from build123d import *

# Parameters (mm, degrees)
BASIC_BOX_OUTLINE_W                                = 108
BASIC_BOX_OUTLINE_H                                = 64
BASIC_BOX_OUTLINE_W_2                              = 98
BASIC_BOX_OUTLINE_H_2                              = 54
SIDE_WALLS_DEPTH                                   = 10
BOTTOM_START                                       = -2
BOTTOM_WALL_OUTLINE_W                              = 98
BOTTOM_WALL_OUTLINE_H                              = 54
BOTTOM_WALL_DEPTH                                  = 2
INNER_WALLS_TO_HOLD_DEVICES_W                      = 2
INNER_WALLS_TO_HOLD_DEVICES_H                      = 16
INSIDE_WALLS_DEPTH                                 = 10
SCREW_HOLES_R                                      = 5
SCREWS_DEPTH                                       = 10
ALIGNMENT_W                                        = 104
ALIGNMENT_H                                        = 60
ALIGNMENT_W_2                                      = 102
ALIGNMENT_H_2                                      = 58
ALIGNMENT_BUMP_DEPTH                               = 2
LEFT_START                                         = -5
LEFT_HOLE_DEPTH                                    = 5
RIGHT_HOLE_DEPTH                                   = 5
SKETCH6_W                                          = 23
SKETCH6_H                                          = 10
CUT_EXTRUDE2_DEPTH                                 = 10
CSK_FOR_10_FLAT_HEAD_MACHINE_SCREW_100_D           = 5.1054
CSK_FOR_10_FLAT_HEAD_MACHINE_SCREW_100_CSINK_D     = 9.779
CSK_FOR_10_FLAT_HEAD_MACHINE_SCREW_100_CSINK_ANGLE = 100
FILLET1_R                                          = 1.5
FILLET2_R                                          = 1.5
FILLET3_R                                          = 1


# Read off the part's stored shape, not the designer's step: bottom wall
with BuildPart() as part:
    # basic box outline → side walls (new body)
    with BuildSketch(Plane(origin=(0, 0, 0), x_dir=(1, 0, 0), z_dir=(0, 1, 0))):
        with Locations((0, 32)):
            Rectangle(BASIC_BOX_OUTLINE_W, BASIC_BOX_OUTLINE_H)
        with Locations((0, 32)):
            Rectangle(BASIC_BOX_OUTLINE_W_2, BASIC_BOX_OUTLINE_H_2, mode=Mode.SUBTRACT)
    extrude(amount=-SIDE_WALLS_DEPTH)

    # bottom wall outline → bottom wall (add)
    with BuildSketch(Plane(origin=(0, 0, 0), x_dir=(1, 0, 0), z_dir=(0, 1, 0)).offset(BOTTOM_START)):
        with Locations((0, 32)):
            Rectangle(BOTTOM_WALL_OUTLINE_W, BOTTOM_WALL_OUTLINE_H)
    extrude(amount=BOTTOM_WALL_DEPTH)

    # inner walls to hold devices → inside walls (add)
    with BuildSketch(Plane(origin=(0, 0, 0), x_dir=(1, 0, 0), z_dir=(0, 1, 0))):
        Polygon((-47, 59), (-49, 59), (-49, 55.5), (-33, 55.5), (-33, 58), (-24, 58), (-24, 54), (-14, 54), (-14, 55), (1, 55), (1, 59), (-1, 59), (-1, 57), (-16, 57), (-16, 56), (-22, 56), (-22, 59), (-35, 59), (-35, 57.5), (-47, 57.5), align=None)
        Polygon((27, 59), (25, 59), (25, 55), (40, 55), (40, 54), (49, 54), (49, 56), (42, 56), (42, 57), (27, 57), align=None)
        Polygon((49, 50), (40, 50), (40, 49), (25, 49), (25, 41), (16, 41), (16, 39), (27, 39), (27, 47), (42, 47), (42, 48), (49, 48), align=None)
        Polygon((-14, 50), (-24, 50), (-24, 46), (-33, 46), (-33, 48.5), (-35, 48.5), (-35, 21), (-33, 21), (-33, 44), (-22, 44), (-22, 48), (-16, 48), (-16, 47), (-1, 47), (-1, 39), (5, 39), (5, 41), (1, 41), (1, 49), (-14, 49), align=None)
        with Locations((-12, 13)):
            Rectangle(INNER_WALLS_TO_HOLD_DEVICES_W, INNER_WALLS_TO_HOLD_DEVICES_H)
    extrude(amount=-INSIDE_WALLS_DEPTH)

    # screw holes → screws (add)
    with BuildSketch(Plane(origin=(0, 0, 0), x_dir=(1, 0, 0), z_dir=(0, 1, 0))):
        with Locations(Location((-19, 39, 0), (0, 0, 270))):
            Circle(SCREW_HOLES_R)
        with Locations(Location((39, 39, 0), (0, 0, 270))):
            Circle(SCREW_HOLES_R)
    extrude(amount=-SCREWS_DEPTH)

    # alignment → alignment bump (add)
    with BuildSketch(Plane(origin=(0, -10, 0), x_dir=(-1, 0, 0), z_dir=(0, -1, 0))):
        with Locations((0, 32)):
            Rectangle(ALIGNMENT_W, ALIGNMENT_H)
        with Locations((0, 32)):
            Rectangle(ALIGNMENT_W_2, ALIGNMENT_H_2, mode=Mode.SUBTRACT)
    extrude(amount=ALIGNMENT_BUMP_DEPTH)

    # hole 1 → left hole (cut)
    with BuildSketch(Plane(origin=(54, 0, 0), x_dir=(0, 0, -1), z_dir=(1, 0, 0)).offset(LEFT_START)):
        with BuildLine():
            Line((46, -10), (46, -12))
            Line((46, -12), (58, -12))
            Line((58, -12), (58, -10))
            ThreePointArc((58, -10), (52, -4), (46, -10))
        make_face()
    extrude(amount=LEFT_HOLE_DEPTH, mode=Mode.SUBTRACT)

    # hole 2 → right hole (cut)
    with BuildSketch(Plane.ZY.offset(54)):
        with BuildLine():
            Line((-58, -10), (-58, -12))
            Line((-58, -12), (-46, -12))
            Line((-46, -12), (-46, -10))
            ThreePointArc((-46, -10), (-52, -4), (-58, -10))
        make_face()
    extrude(amount=-RIGHT_HOLE_DEPTH, mode=Mode.SUBTRACT)

    # Sketch6 → Cut-Extrude2 (cut)
    with BuildSketch(Plane.XY):
        with Locations((-32.5, -7)):
            Rectangle(SKETCH6_W, SKETCH6_H)
    extrude(amount=-CUT_EXTRUDE2_DEPTH, mode=Mode.SUBTRACT)

    # CSK for #10 Flat Head Machine Screw (100)1 (through all)
    with Locations(Plane(origin=(0, 0, 0), x_dir=(1, 0, 0), z_dir=(0, 1, 0))):
        with Locations((-19, 39), (39, 39)):
            CounterSinkHole(CSK_FOR_10_FLAT_HEAD_MACHINE_SCREW_100_D / 2, CSK_FOR_10_FLAT_HEAD_MACHINE_SCREW_100_CSINK_D / 2, counter_sink_angle=CSK_FOR_10_FLAT_HEAD_MACHINE_SCREW_100_CSINK_ANGLE)

    # Fillet1
    fillet1_edges = [part.edges().sort_by_distance(p)[0] for p in [
        (-52, -11, -2),
        (-52, -11, -62),
        (52, -11, -62),
        (52, -11, -2),
        (-51, -11, -61),
        (51, -11, -61),
        (51, -11, -3),
        (-51, -11, -3),
        (-54, -5, -64),
        (54, -5, -64),
        (54, -5, 0),
        (-54, -5, 0),
    ]]
    fillet(fillet1_edges, radius=FILLET1_R)

    # Fillet2
    fillet2_edges = [part.edges().sort_by_distance(p)[0] for p in [
        (0, 0, -64),
        (-54, 0, -32),
        (0, 0, 0),
        (54, 0, -32),
        (-53.560660172, 0, -0.439339828),
        (53.560660172, 0, -0.439339828),
        (53.560660172, 0, -63.560660172),
        (-53.560660172, 0, -63.560660172),
    ]]
    fillet(fillet2_edges, radius=FILLET2_R)

    # Fillet3
    # the kernel refuses this fillet: 1 mm, written as the material it adds along each edge
    with BuildSketch(Plane(origin=(-19, -2, -39), x_dir=(0, 0, 1), z_dir=(-1, 0, 0))) as fillet3_piece_1:
        with BuildLine():
            CenterArc((5 + FILLET3_R, -FILLET3_R), FILLET3_R, 90, 90)
            Line((5, -FILLET3_R), (5, 0))
            Line((5, 0), (5 + FILLET3_R, 0))
        make_face()
    revolve(axis=Axis((-19, -2, -39), (0, 1, 0)))
    with BuildSketch(Plane(origin=(39, -2, -39), x_dir=(0, 0, 1), z_dir=(-1, 0, 0))) as fillet3_piece_2:
        with BuildLine():
            CenterArc((5 + FILLET3_R, -FILLET3_R), FILLET3_R, 90, 90)
            Line((5, -FILLET3_R), (5, 0))
            Line((5, 0), (5 + FILLET3_R, 0))
        make_face()
    revolve(axis=Axis((39, -2, -39), (0, 1, 0)))


solid = part.part
Read the model definition and answer for the solid it produces. Units are mm, in the model's axes. A direction names the side the tool comes from. Give positions to 0.01 mm unless a question says otherwise; leave off trailing zeros. Loops run counter-clockwise (first coordinate to the right, second up) from the corner with the lowest first, then second, coordinate; pieces in that order, holes last. Notation, with made-up numbers: M 19,89 L 60,89 A20 ccw 60,98 Z; hole C 45,87 d5. An arc over 180 degrees is marked long. Write each question's results on one line, items separated by ' | '.
1. Straight lines are drawn through the part: line 1 (Z direction, x = 2, y = -6.75); line 2 (Z direction, x = 33.5, y = -7.5); line 3 (X direction, y = -3.5, z = -26). For each, find the intervals that lie inside material, in ascending order. Write a range as [from, to].
Values:
line 1: z = [-64, -59], [-41, -39], [-5, 0] | line 2: z = [-64, -59], [-57, -55], [-49, -47], [-5, 0] | line 3: x = [-54, -49], [-35, -33], [49, 54]
2. Section C-C on y = -7 is taken. State how many separate pieces and enclosed holes the cut face has, plus the area to 3 significant figures.
Values:
separate pieces: 7 | enclosed holes: 4 | area: 1,950 mm^2
3. The mould has two halves that part along Z. Classify faces 5 (the face through (-51, -11, -25)), 6 (the face through (52, -11, -59)): pulls with the +Z half, pulls with the -Z half, needs draft (parallel to the pull), parting line crosses it, or undercut.
Values:
face 5: undercut | face 6: needs draft
4. Section A-A on z = -26.5 is taken. Give the vertices of the cut face in (x, y).
Values:
outline: M -54,-10 L -52,-10 L -52,-12 L -51,-12 L -51,-10 L -49,-10 L -49,-2 L -35,-2 L -35,-10 L -33,-10 L -33,-2 L 49,-2 L 49,-10 L 51,-10 L 51,-12 L 52,-12 L 52,-10 L 54,-10 L 54,-1.5 A1.5 ccw 52.5,0 L -52.5,0 A1.5 ccw -54,-1.5 Z
5. Section B-B on x = -45.5 is taken. Give the vertices of the cut face in (y, z), plus the area to 3 significant figures.
Values:
outline: M -12,-62 L -10,-62 L -10,-64 L -1.5,-64 A1.5 ccw 0,-62.5 L 0,-1.5 A1.5 ccw -1.5,0 L -10,0 L -10,-2 L -12,-2 L -12,-3 L -10,-3 L -10,-5 L -2,-5 L -2,-55.5 L -10,-55.5 L -10,-57.5 L -2,-57.5 L -2,-59 L -10,-59 L -10,-61 L -12,-61 Z | area: 227 mm^2
6. Given pin 1 (5 mm diameter, centred on x = 42.5, z = -32.5, fed in from -Y); pin 2 (1.5 mm diameter, centred on x = -33, z = -12, fed in from -Y); pin 3 (2 mm diameter, centred on x = -24.5, y = -7.5, fed in from +Z), each flat-ended and moving along its own axis, determine where each tip first touches the part or whether it passes through.
Values:
pin 1: stops at y = -10 | pin 2: stops at y = -2 | pin 3: stops at z = -36.82
7. A tool of negligible diameter and unlimited length cuts with its end or side. For faces 1 (the face through (33, -10, -1)), 2 (the face through (54, -6, -32)), 3 (the face through (-22, -6, -57)), 4 (the face through (-52, -11, -59)), from which of +Z, -Z, +X, -X, +Y, -Y can it reach the whole face along a straight path? Write none if from no direction.
Values:
face 1: +Z, +X, -Y | face 2: +Z, -Z, +X, +Y, -Y | face 3: -Y | face 4: +Z, -Z, -X, -Y
8. Section D-D on z = -52 is taken. Give the vertices of the cut face in (x, y).
Values:
outline: M -54,-4 L -49,-4 L -49,-2 L 49,-2 L 49,-4 L 54,-4 L 54,-1.5 A1.5 ccw 52.5,0 L -52.5,0 A1.5 ccw -54,-1.5 Z
